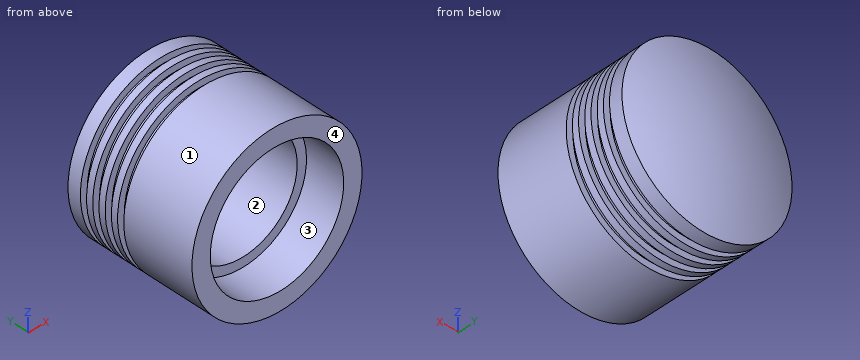
```python
from build123d import *


with BuildPart() as part:
    # Sketch1 → Revolve1 (revolve)
    with BuildSketch(Plane.XY, mode=Mode.PRIVATE) as revolve1_sk:
        with BuildLine():
            Line((63.722275674, 0), (63.722275674, 55))
            Line((63.722275674, 55), (58.722275674, 55))
            Line((58.722275674, 55), (58.722275674, 60))
            Line((58.722275674, 60), (63.722275674, 60))
            Line((63.722275674, 60), (63.722275674, 65))
            Line((63.722275674, 65), (58.722275674, 65))
            Line((58.722275674, 65), (58.722275674, 70))
            Line((58.722275674, 70), (63.722275674, 70))
            Line((63.722275674, 70), (63.722275674, 75))
            Line((63.722275674, 75), (58.722275674, 75))
            Line((58.722275674, 75), (58.722275674, 80))
            Line((58.722275674, 80), (63.722275674, 80))
            Line((63.722275674, 80), (63.722275674, 85))
            Line((63.722275674, 85), (58.722275674, 85))
            Line((58.722275674, 85), (58.722275674, 90))
            Line((58.722275674, 90), (63.722275674, 90))
            Line((63.722275674, 90), (63.722275674, 100))
            ThreePointArc((63.722275674, 100), (32.458256966, 109.267160728), (0, 112.394569945))
            Line((0, 112.394569945), (0, 105.394569945))
            ThreePointArc((0, 105.394569945), (21.692969078, 103.944608919), (43, 99.620522001))
            Line((43, 99.620522001), (43, 30))
            Line((43, 30), (50, 30))
            Line((50, 30), (50, 0))
            Line((50, 0), (63.722275674, 0))
        make_face()
    revolve(revolve1_sk.sketch.rotate(Axis((0, 0, 0), (0, 1, 0)), 90), axis=Axis((0, 0, 0), (0, 1, 0)))


solid = part.part
```
Part model, mm, in its own coordinate system. Face numbers are marked on the shaded views. Give positions to 0.01 mm unless a question says otherwise; leave off trailing zeros. Write each loop counter-clockwise with the first axis right and the second up, starting at its lowest first coordinate (ties: lowest second). Pieces come first, ordered by that corner, then holes. Notation, with made-up numbers: (1, 86.25) -> (13, 86.25) arc R14 ccw to (13, 90.25) -> close; hole circle Ø2 at (31.25, 87.25). An arc over 180 degrees is marked (long way). Put each result on its own line as item: value. Start each with the question number.
Item 1: Pull direction Z, two halves, no side cores. Call the marked faces 1, 2, 3 and 4: pulls with the +Z half, pulls with the -Z half, needs draft (parallel to the pull), parting line crosses it, or undercut.
Item 2: Wall check: L1, parallel to X at y = 74, z = 0; L2, parallel to X at y = 15.75, z = 0; L3, parallel to Z at x = -9, y = 19. Give the ranges that are in metal, low to high. Write a range as [from, to].
Item 3: Pin check, flat tips, straight feed: pin 1 Ø2 at (y, z) = (78.5, -24) entering from -X; pin 2 Ø3 at (x, y) = (-32.5, 74.5) entering from +Z; pin 3 Ø1.5 at (x, y) = (-43, 82.5) entering from -Z. Stop position of each tip, or through.
Item 4: Cut at A-A (y = 41). List the corners of the cut face in (x, z), then the cut area to 3 significant figures.
Answer list:
1. face 1: parting line crosses it
1. face 2: undercut
1. face 3: undercut
1. face 4: needs draft
2. L1: x = [-63.72, -43], [43, 63.72]
2. L2: x = [-63.72, -50], [50, 63.72]
2. L3: z = [-63.08, -49.18], [49.18, 63.08]
3. pin 1: stops at x = -54.03
3. pin 2: stops at z = 55.67
3. pin 3: stops at z = -47.7
4. outline: circle Ø127.44 at (0, 0); hole circle Ø86 at (0, 0)
4. area: 6,950 mm2
